The listing builds one solid part. Answer for the finished solid, in the listing's coordinates (mm). Round coordinates to 2 decimals unless told otherwise and drop trailing zeros. Write each loop counter-clockwise with the first axis right and the second up, starting at its lowest first coordinate (ties: lowest second). Pieces come first, ordered by that corner, then holes.
(1) The mould has two halves that part along Z. Classify faces 1 (the face through (23, 0, -13)), 2 (the face through (-1, -1.5, 0)), 3 (the face through (-1, 0, -21)): +Z half, -Z half, draft (parallel to the pull), parting line (faces both ways), or undercut.
(2) Each of these flat-tipped pins is pushed along its axis until it touches: pin 1 Ø3.5 at (x, z) = (-21, -13) entering from -Y; pin 2 Ø1 at (y, z) = (1, 12.5) entering from +X; pin 3 Ø1 at (y, z) = (-1, 5) entering from -X. Where does it stop, or does it pass through?
(3) A cutting plane is placed at B-B, the plane z = 13. Give the vertices of the cut face in (x, y), and give its area (3 significant figures).
(4) Find the intervals of material crossed by probe 1 along Z at (x, y) = (-67.5, 0.6); probe 2 along X at (y, z) = (1.35, -13.5); probe 3 along X at (y, z) = (0.75, 13), in increasing order.
(5) A cutting plane is placed at A-A, the plane y = 0.6. Give the number of separate pieces and of enclosed holes in the cut face, and give its area (3 significant figures).
from build123d import *

# Parameters (mm, degrees)
SKETCH_1_W          = 180
SKETCH_1_H          = 3
EXTRUDE_1_DEPTH     = 21
SKETCH_2_R          = 2
CUT_EXTRUDE_1_DEPTH = 93.466210045
SKETCH_3_R          = 1.05
CUT_EXTRUDE_2_DEPTH = 93.466210045
FILLET_1_R          = 21


with BuildPart() as part:
    # 草图1 → 凸台-拉伸1 (new, symmetric)
    with BuildSketch(Plane.XY):
        Rectangle(SKETCH_1_W, SKETCH_1_H)
    extrude(amount=EXTRUDE_1_DEPTH, both=True)

    # 草图2 → 切除-拉伸1 (cut, through all)
    with BuildSketch(Plane(origin=(0, 1.5, 0), x_dir=(1, 0, 0), z_dir=(0, 1, 0))):
        with Locations(Location((-21, 13, 0), (0, 0, 270))):
            Circle(SKETCH_2_R)
        with Locations(Location((21, 13, 0), (0, 0, 270))):
            Circle(SKETCH_2_R)
        with Locations(Location((21, -13, 0), (0, 0, 270))):
            Circle(SKETCH_2_R)
        with Locations(Location((-21, -13, 0), (0, 0, 270))):
            Circle(SKETCH_2_R)
    extrude(amount=-CUT_EXTRUDE_1_DEPTH, mode=Mode.SUBTRACT)

    # 草图3 → 切除-拉伸2 (cut, through all)
    with BuildSketch(Plane(origin=(0, 1.5, 0), x_dir=(1, 0, 0), z_dir=(0, 1, 0))):
        with Locations(Location((55, 9.5, 0), (0, 0, 270))):
            Circle(SKETCH_3_R)
        with Locations(Location((55, -9.5, 0), (0, 0, 270))):
            Circle(SKETCH_3_R)
        with Locations(Location((42.5, 0, 0), (0, 0, 270))):
            Circle(SKETCH_3_R)
        with Locations(Location((67.5, 0, 0), (0, 0, 270))):
            Circle(SKETCH_3_R)
    cut_extrude_2 = extrude(amount=-CUT_EXTRUDE_2_DEPTH, mode=Mode.SUBTRACT)

    # 镜向1: 切除-拉伸2 across plane
    add(cut_extrude_2.mirror(Plane(origin=(0, 0, 0), x_dir=(0, 0, 1), z_dir=(1, 0, 0))), mode=Mode.SUBTRACT)

    # 圆角1
    fillet_1_edges = [part.edges().sort_by_distance(p)[0] for p in [
        (90, 0, 21),
        (-90, 0, 21),
        (-90, 0, -21),
        (90, 0, -21),
    ]]
    fillet(fillet_1_edges, radius=FILLET_1_R - 0.0001)  # a hair under: the kernel refuses the full size


solid = part.part
Solutions:
1. face 1: undercut
1. face 2: draft
1. face 3: -Z half
2. pin 1: passes through
2. pin 2: stops at x = 86.23
2. pin 3: stops at x = -89.51
3. outline: (-85.49, -1.5) - (-23, -1.5) - (-23, 1.5) - (-85.49, 1.5) - close; (-19, -1.5) - (19, -1.5) - (19, 1.5) - (-19, 1.5) - close; (23, -1.5) - (85.49, -1.5) - (85.49, 1.5) - (23, 1.5) - close
3. area: 489 mm2
4. probe 1: z = -21 to -1.05, 1.05 to 21
4. probe 2: x = -85.09 to -22.94, -19.06 to 19.06, 22.94 to 85.09
4. probe 3: x = -85.49 to -23, -19 to 19, 23 to 85.49
5. separate pieces: 1
5. enclosed holes: 12
5. area: 7,100 mm2
